```python
from build123d import *

# Parameters (mm, degrees)
BOSS_EXTRUDE1_DEPTH = 7
SKETCH1_3_W         = 7.858578644
SKETCH1_3_H         = 0.8
BOSS_EXTRUDE2_DEPTH = 3.5


with BuildPart() as part:
    # Sketch1 → Boss-Extrude1 (new body)
    with BuildSketch(Plane(origin=(0, 0, 0), x_dir=(0, 0, -1), z_dir=(1, 0, 0))):
        Polygon((-14.9, 4.6), (-7.041421356, 4.6), (-7.041421356, 1.6), (-5.041421356, 1.6), (-2.041421356, 4.6), (-0.55, 4.6), (-0.55, 2.3), (-2.05, 2.3), (-2.05, 1.2), (2.05, 1.2), (2.05, 2.3), (0.55, 2.3), (0.55, 4.6), (2.041421356, 4.6), (5.041421356, 1.6), (7.041421356, 1.6), (7.041421356, 4.6), (14.9, 4.6), (14.9, 1.6), (18.4, 1.6), (18.4, 2.4), (16.9, 2.4), (16.9, 6.1), (-16.9, 6.1), (-16.9, 2.4), (-18.4, 2.4), (-18.4, 1.6), (-14.9, 1.6), align=None)
    extrude(amount=BOSS_EXTRUDE1_DEPTH)

    # Sketch1<3> → Boss-Extrude2 (add, symmetric)
    with BuildSketch(Plane(origin=(0, 0, 0), x_dir=(0, 0, -1), z_dir=(1, 0, 0))):
        Polygon((7.041421356, 2.4), (4.241421356, 2.4), (5.041421356, 1.6), (7.041421356, 1.6), align=None)
        Polygon((17, 2.4), (16.9, 2.4), (14.9, 2.4), (14.9, 1.6), (17, 1.6), (18.4, 1.6), (18.4, 2.4), align=None)
        with Locations((10.970710678, 2)):
            Rectangle(SKETCH1_3_W, SKETCH1_3_H)
        with Locations((-10.970710678, 2)):
            Rectangle(SKETCH1_3_W, SKETCH1_3_H)
        Polygon((-4.241421356, 2.4), (-7.041421356, 2.4), (-7.041421356, 1.6), (-5.041421356, 1.6), align=None)
        Polygon((-14.9, 1.6), (-14.9, 2.4), (-16.9, 2.4), (-17, 2.4), (-18.4, 2.4), (-18.4, 1.6), (-17, 1.6), align=None)
    extrude(amount=BOSS_EXTRUDE2_DEPTH, both=True)


solid = part.part
```
Can you work these out from the model? Positions are in its coordinate system, mm. A direction names the side the tool comes from. Round coordinates to 2 decimals unless told otherwise and drop trailing zeros. Loops run counter-clockwise (first coordinate to the right, second up) from the corner with the lowest first, then second, coordinate; pieces in that order, holes last.
Item 1: Suppose I cut it at A-A, the plane z = 8. Write out the boundary of the cut face in (x, y).
Item 2: Will these pins go through, and if not, where does the flat tip stop? pin 1 Ø2 at (x, y) = (2.5, 4) entering from -Z; pin 2 Ø3 at (x, z) = (1.5, 12.5) entering from -Y; pin 3 Ø1.5 at (x, y) = (2, 3.5) entering from +Z; pin 4 Ø2.5 at (x, y) = (4, 3.5) entering from -Z.
Item 3: If we mould it in two halves opening along Z, with no side actions, what happens to faces 5 (the flat face through (1, 1.6, 12)), 6 (the flat face through (3, 4, -16.9)), 7 (the flat face through (3, 4.6, 11))? For each: +Z half, -Z half, draft (parallel to the pull), parting line (faces both ways), or undercut.
Item 4: Please list where these lines run through material, in increasing order: L1, parallel to Y at x = 2.75, z = 12.5; L2, parallel to Z at x = 1.5, y = 4.2; L3, parallel to Z at x = 2.5, y = 2.8.
Item 5: Which directions (+Z, -Z, +X, -X, +Y, -Y) give clear straight access to the entire face, cutting with the end or side of a thin tool? Please do faces 1 (the flat face through (3, 2, 2.05)), 2 (the flat face through (1, 2.4, 11)), 3 (the flat face through (3, 4.6, -1)), 4 (the flat face through (1, 1.6, -12)).
Item 6: Suppose I cut it at B-B, the plane y = 3.1. Write out the boundary of the cut face in (x, z).
Item 7: Suppose I cut it at D-D, the plane x = -1.25. Write out the boundary of the cut face in (y, z).
Item 8: Suppose I cut it at C-C, the plane x = 2.75. Write out the boundary of the cut face in (y, z).
Reported:
1. outline: (-3.5, 1.6) - (3.5, 1.6) - (3.5, 2.4) - (-3.5, 2.4) - close; (0, 4.6) - (7, 4.6) - (7, 6.1) - (0, 6.1) - close
2. pin 1: stops at z = -16.9
2. pin 2: stops at y = 1.6
2. pin 3: stops at z = 16.9
2. pin 4: stops at z = -18.4
3. face 5: draft
3. face 6: -Z half
3. face 7: undercut
4. L1: y = 1.6 to 2.4, 4.6 to 6.1
4. L2: z = -16.9 to -14.9, -7.04 to -2.44, -0.55 to 0.55, 2.44 to 7.04, 14.9 to 16.9
4. L3: z = -16.9 to -14.9, -7.04 to -3.84, -0.55 to 0.55, 3.84 to 7.04, 14.9 to 16.9
5. face 1: +X, -X, -Y
5. face 2: -X
5. face 3: +X, -X
5. face 4: -Z, +X, -X, -Y
6. outline: (0, -16.9) - (7, -16.9) - (7, -14.9) - (0, -14.9) - close; (0, -7.04) - (7, -7.04) - (7, -3.54) - (0, -3.54) - close; (0, -0.55) - (7, -0.55) - (7, 0.55) - (0, 0.55) - close; (0, 3.54) - (7, 3.54) - (7, 7.04) - (0, 7.04) - close; (0, 14.9) - (7, 14.9) - (7, 16.9) - (0, 16.9) - close
7. outline: (1.6, -18.4) - (2.4, -18.4) - (2.4, -4.24) - (1.6, -5.04) - close; (1.6, 5.04) - (2.4, 4.24) - (2.4, 18.4) - (1.6, 18.4) - close
8. outline: (1.2, -2.05) - (2.3, -2.05) - (2.3, -0.55) - (4.6, -0.55) - (4.6, -2.04) - (1.6, -5.04) - (1.6, -18.4) - (2.4, -18.4) - (2.4, -16.9) - (6.1, -16.9) - (6.1, 16.9) - (2.4, 16.9) - (2.4, 18.4) - (1.6, 18.4) - (1.6, 5.04) - (4.6, 2.04) - (4.6, 0.55) - (2.3, 0.55) - (2.3, 2.05) - (1.2, 2.05) - close; hole (2.4, -14.9) - (4.6, -14.9) - (4.6, -7.04) - (2.4, -7.04) - close; hole (2.4, 7.04) - (4.6, 7.04) - (4.6, 14.9) - (2.4, 14.9) - close
